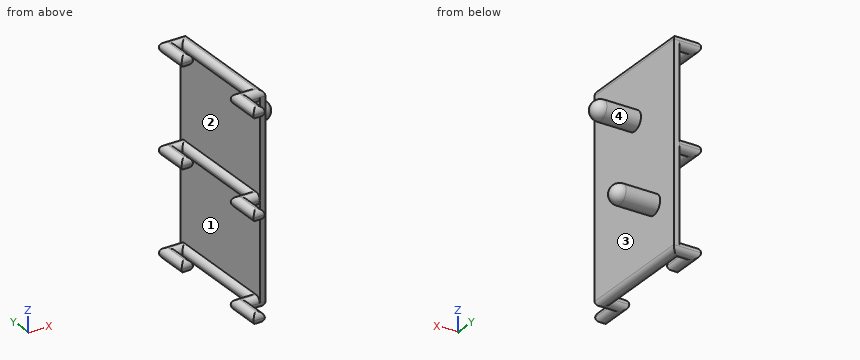
from build123d import *

# Parameters (mm, degrees)
EXTRU_MINCE1_DEPTH           = 2.3
CONG_1_R                     = 2.3
ESQUISSE2_W                  = 80
ESQUISSE2_H                  = 49.6
BOSS_EXTRU_1_DEPTH           = 2.3
R_P_TITION_START             = 77.7
R_P_TITION_LIN_AIRE1_DEPTH   = 4.6
R_P_TITION_START_2           = 37.7
R_P_TITION_LIN_AIRE1_2_DEPTH = 4.6
CONG_2_R                     = 2.3
ESQUISSE3_R                  = 4
BOSS_EXTRU_2_DEPTH           = 18
CONG_3_R                     = 4


# Read off the part's stored shape, not the designer's step: Répétition linéaire1
with BuildPart() as part:
    # Esquisse1 → Extru.-Mince1 (new, symmetric)
    with BuildSketch(Plane.XY):
        Polygon((-4.3, -57), (-4.3, -47.3), (2.3, -47.3), (2.3, 2.3), (-8.9, 2.3), (-8.9, -12), (-4.3, -12), (-4.3, -2.3), (-2.3, -2.3), (-2.3, -42.7), (-8.9, -42.7), (-8.9, -57), align=None)
    extrude(amount=EXTRU_MINCE1_DEPTH, both=True)

    # Congé1
    cong_1_edges = [part.edges().sort_by_distance(p)[0] for p in [
        (-6.6, -57, -2.3),
        (-4.3, -52.15, -2.3),
        (-1, -47.3, -2.3),
        (2.3, -22.5, -2.3),
        (-3.3, 2.3, -2.3),
        (-8.9, -4.85, -2.3),
        (-6.6, -12, -2.3),
        (-4.3, -7.15, -2.3),
        (-3.3, -2.3, -2.3),
        (-2.3, -22.5, -2.3),
        (-5.6, -42.7, -2.3),
        (-8.9, -49.85, -2.3),
        (-5.6, -42.7, 2.3),
        (-2.3, -22.5, 2.3),
        (-3.3, -2.3, 2.3),
        (-4.3, -7.15, 2.3),
        (-6.6, -12, 2.3),
        (-8.9, -4.85, 2.3),
        (-3.3, 2.3, 2.3),
        (2.3, -22.5, 2.3),
        (-1, -47.3, 2.3),
        (-4.3, -52.15, 2.3),
        (-6.6, -57, 2.3),
        (-8.9, -49.85, 2.3),
    ]]
    fillet(cong_1_edges, radius=CONG_1_R - 0.0001)  # a hair under: the kernel refuses the full size

    # Esquisse2 → Boss.-Extru.1 (add)
    with BuildSketch(Plane(origin=(0, 0, 0), x_dir=(0, 0, -1), z_dir=(1, 0, 0))):
        with Locations((-40, -22.5)):
            Rectangle(ESQUISSE2_W, ESQUISSE2_H)
    extrude(amount=BOSS_EXTRU_1_DEPTH)

    # Répétition linéaire1 outline → Répétition linéaire1 (add)
    with BuildSketch(Plane.XY.offset(R_P_TITION_START)):
        Polygon((-8.9, 2.3), (-8.9, -12), (-4.3, -12), (-4.3, -2.3), (-2.3, -2.3), (-2.3, -42.7), (-8.9, -42.7), (-8.9, -57), (-4.3, -57), (-4.3, -47.3), (2.3, -47.3), (2.3, 2.3), align=None)
    extrude(amount=R_P_TITION_LIN_AIRE1_DEPTH)

    # R_p_tition lin_aire1 2 outline → R_p_tition lin_aire1 2 (add)
    with BuildSketch(Plane.XY.offset(R_P_TITION_START_2)):
        Polygon((0, 2.3), (-8.9, 2.3), (-8.9, -12), (-4.3, -12), (-4.3, -2.3), (-2.3, -2.3), (-2.3, -42.7), (-8.9, -42.7), (-8.9, -57), (-4.3, -57), (-4.3, -47.3), (0, -47.3), align=None)
    extrude(amount=R_P_TITION_LIN_AIRE1_2_DEPTH)

    # Congé2
    cong_2_edges = [part.edges().sort_by_distance(p)[0] for p in [
        (-5.6, -42.7, 42.3),
        (-2.3, -22.5, 42.3),
        (-3.3, -2.3, 42.3),
        (-4.3, -7.15, 42.3),
        (-6.6, -12, 42.3),
        (-8.9, -4.85, 42.3),
        (-4.45, 2.3, 42.3),
        (-2.15, -47.3, 42.3),
        (-4.3, -52.15, 42.3),
        (-6.6, -57, 42.3),
        (-8.9, -49.85, 42.3),
        (-2.15, -47.3, 37.7),
        (-4.3, -52.15, 37.7),
        (-6.6, -57, 37.7),
        (-8.9, -49.85, 37.7),
        (-5.6, -42.7, 37.7),
        (-2.3, -22.5, 37.7),
        (-3.3, -2.3, 37.7),
        (-4.3, -7.15, 37.7),
        (-6.6, -12, 37.7),
        (-8.9, -4.85, 37.7),
        (-4.45, 2.3, 37.7),
        (-5.6, -42.7, 82.3),
        (-2.3, -22.5, 82.3),
        (-3.3, -2.3, 82.3),
        (-4.3, -7.15, 82.3),
        (-6.6, -12, 82.3),
        (-8.9, -4.85, 82.3),
        (-3.3, 2.3, 82.3),
        (2.3, -22.5, 82.3),
        (-1, -47.3, 82.3),
        (-4.3, -52.15, 82.3),
        (-6.6, -57, 82.3),
        (-8.9, -49.85, 82.3),
        (-2.15, -47.3, 77.7),
        (-4.3, -52.15, 77.7),
        (-6.6, -57, 77.7),
        (-8.9, -49.85, 77.7),
        (-5.6, -42.7, 77.7),
        (-2.3, -22.5, 77.7),
        (-3.3, -2.3, 77.7),
        (-4.3, -7.15, 77.7),
        (-6.6, -12, 77.7),
        (-8.9, -4.85, 77.7),
        (-4.45, 2.3, 77.7),
    ]]
    fillet(cong_2_edges, radius=CONG_2_R - 0.0001)  # a hair under: the kernel refuses the full size

    # Esquisse3 → Boss.-Extru.2 (add)
    with BuildSketch(Plane(origin=(2.3, 0, 0), x_dir=(0, 0, -1), z_dir=(1, 0, 0))):
        with Locations((-59, -22.3)):
            Circle(ESQUISSE3_R)
        with Locations((-21, -10.3)):
            Circle(ESQUISSE3_R)
    extrude(amount=BOSS_EXTRU_2_DEPTH)

    # Congé3
    cong_3_edges = [part.edges().sort_by_distance(p)[0] for p in [
        (20.3, -22.3, 63),
        (20.3, -10.3, 25),
    ]]
    fillet(cong_3_edges, radius=CONG_3_R)


solid = part.part
Work out the finished part from the listing and answer in its coordinate system (mm). Face numbers are marked on the shaded views. Give positions to 0.01 mm unless a question says otherwise; leave off trailing zeros. Order: outer loops, then holes, each group sorted by start corner. A loop starts at its lowest first (then second) coordinate and runs counter-clockwise, first axis right, second up. Notation, with made-up numbers: (-6, -9.5) -> (52, -9.5) arc R8 ccw to (52, -4.5) -> close; hole circle Ø8 at (-37.5, 63.25). An arc over 180 degrees is marked (long way). Answer as a JSON object with one key per item and string values. Group by question number.
1. Section B-B on z = 21 is taken. Determine the outline of the cut face in (x, y).
2. Flat-ended cylindrical pins translate along their axes: pin 1 Ø10 at (y, z) = (-35.5, 7) entering from -X; pin 2 Ø25 at (y, z) = (-31.5, 59.5) entering from +X; pin 3 Ø3 at (x, z) = (17.5, 28) entering from +Y; pin 4 Ø5 at (y, z) = (-12, 34.5) entering from -X. Find the tip coordinate at first contact, or state that the pin passes through.
3. Section D-D on x = 8.25 is taken. Determine the outline of the cut face in (y, z), plus the area to 3 significant figures.
4. Consider line 1 along X through (y, z) = (-11.5, 5); line 2 along Z through (x, y) = (-6.25, -52); line 3 along Y through (x, z) = (-6, 78.5). Determine where each line is inside the solid, lowest interval first. Write a range as [from, to].
5. Section C-C on x = 1.25 is taken. Determine the outline of the cut face in (y, z), plus the area to 3 significant figures.
6. The mould has two halves that part along Z. Classify the marked faces 1, 2, 3 and 4: released by +Z, released by -Z, zero draft, split by the parting line, or undercut.
Result sheet:
{
 "1": {"outline": "(0, -47.3) -> (2.3, -47.3) -> (2.3, -14.3) -> (16.3, -14.3) arc R4 ccw to (16.3, -6.3) -> (2.3, -6.3) -> (2.3, 2.3) -> (0, 2.3) -> close"},
 "2": {"pin 1": "stops at x = -1.14", "pin 2": "stops at x = 20.3", "pin 3": "passes through", "pin 4": "stops at x = 0"},
 "3": {"outline": "circle Ø8 at (-22.3, 59); circle Ø8 at (-10.3, 21)", "area": "101 mm^2"},
 "4": {"line 1": "x = [0, 2.3]", "line 2": "z = [-2.27, 2.27], [37.73, 42.27], [77.73, 82.27]", "line 3": "y = [-56.44, -43.26], [-11.44, 1.74]"},
 "5": {"outline": "(-47.3, 0) arc R2.3 ccw to (-46.25, -1.93) -> (1.25, -1.93) arc R2.3 ccw to (2.3, 0) -> (2.3, 80) arc R2.3 ccw to (1.25, 81.93) -> (-46.25, 81.93) arc R2.3 ccw to (-47.3, 80) -> close", "area": "4,160 mm^2"},
 "6": {"face 1": "undercut", "face 2": "undercut", "face 3": "zero draft", "face 4": "split by the parting line"}
}
